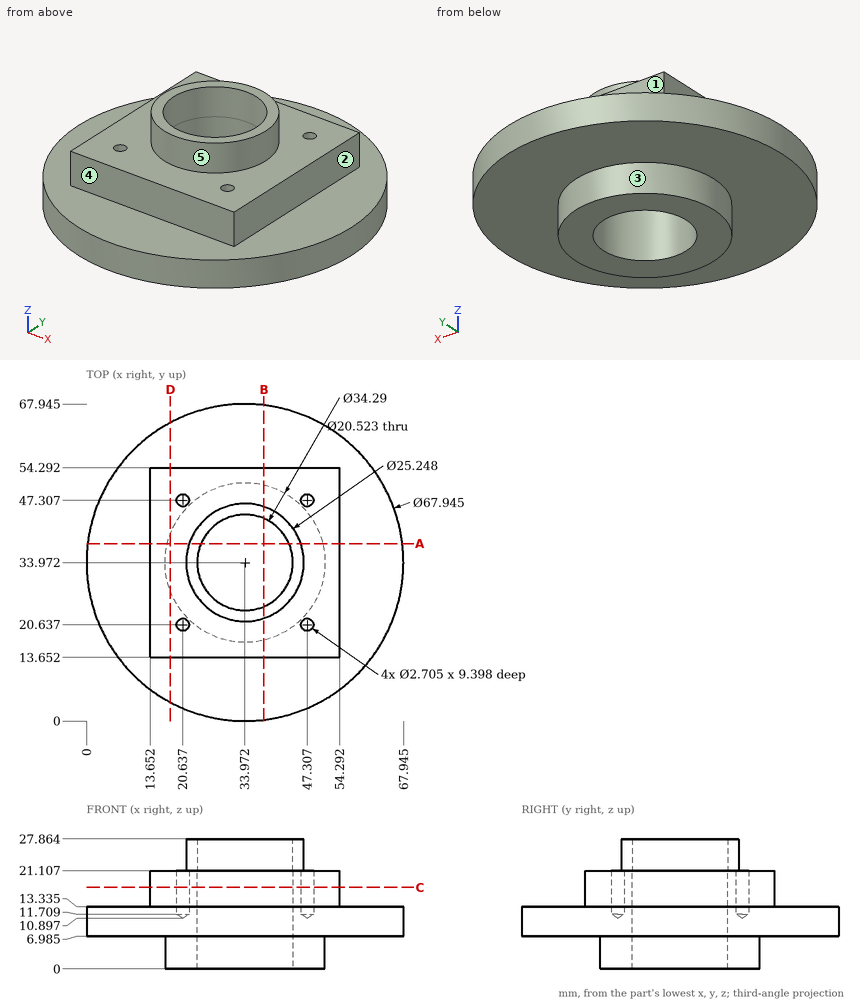
The drawing under review shows one solid part. Ordinate dimensions are in mm from its lowest x, y, z. A direction names the side the tool comes from. Round coordinates to 2 decimals unless told otherwise and drop trailing zeros. Write each loop counter-clockwise with the first axis right and the second up, starting at its lowest first coordinate (ties: lowest second). Pieces come first, ordered by that corner, then holes. Notation, with made-up numbers: M 77,-20 L 122,-20 A22 cw 122,7 Z; hole C 86.5,33 d3. An arc over 180 degrees is marked long. One line per item, written item: value. Start each with the question number.
(1) Wall thickness on line 1 (Z direction, x = 6, y = 17) (1 decimal); line 2 (Z direction, x = 30, y = 15) (1 decimal); line 3 (Y direction, x = 38.5, z = 13.5) (1 decimal): over which ranges is each line inside the solid? List them lowest first.
(2) We need section D-D (x = 18). Give the boundary of the cut face in (y, z) (1 decimal).
(3) We need section C-C (z = 17.5). Give the boundary of the cut face in (x, y) (1 decimal), and give its area (3 significant figures).
(4) We need section A-A (y = 38). Give the boundary of the cut face in (x, z) (1 decimal), and give its area (3 significant figures).
(5) Insertion check: pin 1 (1.6 mm diameter, centred on x = 20.64, y = 20.64, fed in from +Z); pin 2 (3 mm diameter, centred on x = 35.5, z = 13.5, fed in from +Y) (1 decimal); pin 3 (2 mm diameter, centred on x = 47.31, y = 20.64, fed in from +Z). Each pin has a flat end and moves straight along its axis. Give the tip position at first contact, or say it passes through.
(6) Machinability: for the marked faces 1, 2, 3, 4 and 5, which of the approach directions +Z, -Z, +X, -X, +Y, -Y give a long, thin tool a straight path to every point of the face, cutting with its end or side? Answer none if there is none.
Result:
1. line 1: 7 to 13.3
1. line 2: 7 to 21.1
1. line 3: 13.7 to 24.8, 43.2 to 54.3
2. outline: M 4,7 L 27.7,7 L 27.7,0 L 40.2,0 L 40.2,7 L 64,7 L 64,13.3 L 54.3,13.3 L 54.3,21.1 L 13.7,21.1 L 13.7,13.3 L 4,13.3 Z
3. outline: M 13.7,13.7 L 54.3,13.7 L 54.3,54.3 L 13.7,54.3 Z; hole C 20.6,20.6 d2.7; hole C 20.6,47.3 d2.7; hole C 34,34 d20.5; hole C 47.3,20.6 d2.7; hole C 47.3,47.3 d2.7
3. area: 1,300 mm²
4. outline: M 0.2,7 L 17.3,7 L 17.3,0 L 24.5,0 L 24.5,27.9 L 22,27.9 L 22,21.1 L 13.7,21.1 L 13.7,13.3 L 0.2,13.3 Z; M 43.4,0 L 50.6,0 L 50.6,7 L 67.7,7 L 67.7,13.3 L 54.3,13.3 L 54.3,21.1 L 45.9,21.1 L 45.9,27.9 L 43.4,27.9 Z
4. area: 613 mm²
5. pin 1: z = 11.38
5. pin 2: y = 67.9
5. pin 3: z = 11.5
6. face 1: +Z, +X, -X, +Y
6. face 2: +Z, +X, +Y, -Y
6. face 3: -Z
6. face 4: +Z, +X, -X, -Y
6. face 5: +Z
